from build123d import *

# Parameters (mm, degrees)
SKETCH1_W                = 457.2
SKETCH1_H                = 609.6
BOSS_EXTRUDE2_DEPTH      = 6.35
CUT_EXTRUDE1_REACH       = 764.026
SKETCH2_W                = 63.5
SKETCH2_H                = 68.58
SKETCH3_W                = 73.66
SKETCH3_H                = 27.94
CUT_EXTRUDE2_DEPTH       = 63.5
CUT_EXTRUDE4_DEPTH       = 763.026457874
CUT_EXTRUDE4_DEPTH_BACK  = 763.026457874
SKETCH5_W                = 5.08
SKETCH5_H                = 27.94
CUT_EXTRUDE5_DEPTH       = 763.026457874
CUT_EXTRUDE5_DEPTH_BACK  = 763.026457874
CUT_EXTRUDE6_DEPTH       = 763.026457874
CUT_EXTRUDE6_DEPTH_BACK  = 763.026457874
SKETCH7_W                = 12.7
SKETCH7_H                = 355.6
CUT_EXTRUDE8_START       = -6.35
CUT_EXTRUDE8_OUTLINE_W   = 6.35
CUT_EXTRUDE8_OUTLINE_H   = 127
CUT_EXTRUDE8_DEPTH       = 6.35
CUT_EXTRUDE9_DEPTH       = 763.026457874
CUT_EXTRUDE9_DEPTH_BACK  = 763.026457874
CUT_EXTRUDE10_START      = -6.35
CUT_EXTRUDE10_OUTLINE_W  = 6.35
CUT_EXTRUDE10_OUTLINE_H  = 127
CUT_EXTRUDE10_DEPTH      = 6.35
CUT_EXTRUDE11_DEPTH      = 759.233608461
CUT_EXTRUDE11_DEPTH_BACK = 759.233608461
CUT_EXTRUDE12_DEPTH      = 759.233608461
CUT_EXTRUDE12_DEPTH_BACK = 759.233608461
SKETCH4_R                = 6.4135
CUT_EXTRUDE13_DEPTH      = 759.233608461


# Read off the part's stored shape, not the designer's step: Cut-Extrude8, Cut-Extrude10
with BuildPart() as part:
    # Sketch1 → Boss-Extrude2 (new body)
    with BuildSketch(Plane.XY):
        with Locations((-228.6, 304.8)):
            Rectangle(SKETCH1_W, SKETCH1_H)
    extrude(amount=BOSS_EXTRUDE2_DEPTH)

    # Sketch2 → Cut-Extrude1 (cut, up to next)
    with BuildSketch(Plane.XY.offset(6.35), mode=Mode.PRIVATE) as cut_extrude1_sk1:
        with Locations((-111.175624359, 248.287614127)):
            Rectangle(SKETCH2_W, SKETCH2_H)
    cut_extrude1_tool1 = extrude(cut_extrude1_sk1.sketch, amount=-CUT_EXTRUDE1_REACH, mode=Mode.PRIVATE) & part.part
    add(cut_extrude1_tool1.solids().sort_by_distance((-111.175624, 248.287614, 6.35))[0], mode=Mode.SUBTRACT)

    # Sketch3 → Cut-Extrude2 (cut)
    with BuildSketch(Plane.XY.offset(6.35)):
        with Locations((-115.023623847, 327.440976048)):
            Rectangle(SKETCH3_W, SKETCH3_H)
    extrude(amount=-CUT_EXTRUDE2_DEPTH, mode=Mode.SUBTRACT)

    # Sketch5 → Cut-Extrude4 (cut, two sides: drawn at the far end of the back side and taken through both)
    with BuildSketch(Plane.XY.offset(6.35).offset(-CUT_EXTRUDE4_DEPTH_BACK)):
        with Locations((-75.653623847, 327.440976048)):
            Rectangle(SKETCH5_W, SKETCH5_H)
    extrude(amount=CUT_EXTRUDE4_DEPTH + CUT_EXTRUDE4_DEPTH_BACK, mode=Mode.SUBTRACT)

    # Sketch6 → Cut-Extrude5 (cut, two sides: drawn at the far end of the back side and taken through both)
    with BuildSketch(Plane.XY.offset(6.35).offset(-CUT_EXTRUDE5_DEPTH_BACK)):
        Polygon((-1796.763236556, 127), (-457.2, 127), (-444.5, 127), (-444.5, 482.6), (-457.2, 482.6), (-1796.763236556, 482.6), (-4475.889709667, 482.6), (-4475.889709667, 127), align=None)
    extrude(amount=CUT_EXTRUDE5_DEPTH + CUT_EXTRUDE5_DEPTH_BACK, mode=Mode.SUBTRACT)

    # Sketch7 → Cut-Extrude6 (cut, two sides: drawn at the far end of the back side and taken through both)
    with BuildSketch(Plane.XY.offset(6.35).offset(-CUT_EXTRUDE6_DEPTH_BACK)):
        with Locations((-6.35, 304.8)):
            Rectangle(SKETCH7_W, SKETCH7_H)
    extrude(amount=CUT_EXTRUDE6_DEPTH + CUT_EXTRUDE6_DEPTH_BACK, mode=Mode.SUBTRACT)

    # Cut-Extrude8 outline → Cut-Extrude8 (cut)
    with BuildSketch(Plane.XY.offset(6.35).offset(CUT_EXTRUDE8_START)):
        with Locations((-454.025, 63.5)):
            Rectangle(CUT_EXTRUDE8_OUTLINE_W, CUT_EXTRUDE8_OUTLINE_H)
    extrude(amount=CUT_EXTRUDE8_DEPTH, mode=Mode.SUBTRACT)

    # Sketch13 → Cut-Extrude9 (cut, two sides: drawn at the far end of the back side and taken through both)
    with BuildSketch(Plane.XY.offset(6.35).offset(-CUT_EXTRUDE9_DEPTH_BACK)):
        Polygon((-450.85, 2136.014036469), (-450.85, 609.6), (-450.85, 482.6), (-450.85, -1043.814036469), (-3503.678072938, -1043.814036469), (-3503.678072938, 2136.014036469), align=None)
    extrude(amount=CUT_EXTRUDE9_DEPTH + CUT_EXTRUDE9_DEPTH_BACK, mode=Mode.SUBTRACT)

    # Cut-Extrude10 outline → Cut-Extrude10 (cut)
    with BuildSketch(Plane.XY.offset(6.35).offset(CUT_EXTRUDE10_START)):
        with Locations((-3.175, 546.1)):
            Rectangle(CUT_EXTRUDE10_OUTLINE_W, CUT_EXTRUDE10_OUTLINE_H)
    extrude(amount=CUT_EXTRUDE10_DEPTH, mode=Mode.SUBTRACT)

    # Sketch16 → Cut-Extrude11 (cut, two sides: drawn at the far end of the back side and taken through both)
    with BuildSketch(Plane.XY.offset(6.35).offset(-CUT_EXTRUDE11_DEPTH_BACK)):
        Polygon((-6.35, 1645.896828812), (-6.35, 127), (-6.35, 0), (-6.35, -1518.896828812), (3031.443657625, -1518.896828812), (3031.443657625, 1645.896828812), align=None)
    extrude(amount=CUT_EXTRUDE11_DEPTH + CUT_EXTRUDE11_DEPTH_BACK, mode=Mode.SUBTRACT)

    # Sketch9 → Cut-Extrude12 (cut, two sides: drawn at the far end of the back side and taken through both)
    with BuildSketch(Plane.XY.offset(6.35).offset(-CUT_EXTRUDE12_DEPTH_BACK)):
        Polygon((-171.45, -1351.158484296), (-171.45, 0), (-171.45, 6.35), (-285.75, 6.35), (-285.75, 0), (-285.75, -1351.158484296), (-285.75, -4053.475452889), (-171.45, -4053.475452889), align=None)
    extrude(amount=CUT_EXTRUDE12_DEPTH + CUT_EXTRUDE12_DEPTH_BACK, mode=Mode.SUBTRACT)

    # Sketch4 → Cut-Extrude13 (cut, through all)
    with BuildSketch(Plane.XY.offset(6.35)):
        with Locations((-292.1, 516.89)):
            Circle(SKETCH4_R)
    extrude(amount=-CUT_EXTRUDE13_DEPTH, mode=Mode.SUBTRACT)


solid = part.part
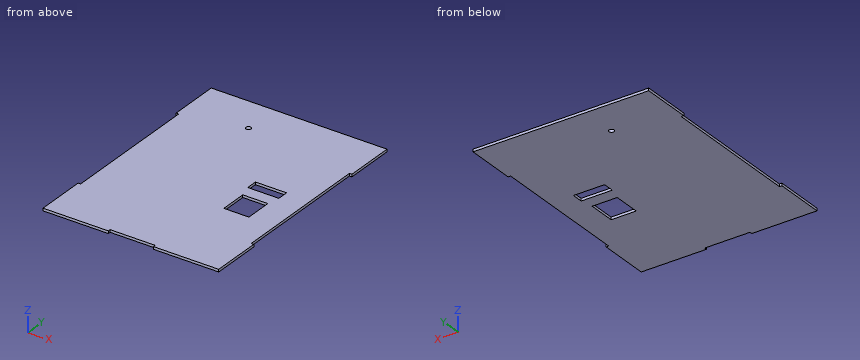
Check sheet for the modelled part. Datum: model origin and axes. Units: mm. Give positions to 0.01 mm unless a question says otherwise; leave off trailing zeros. Loops run counter-clockwise (first coordinate to the right, second up) from the corner with the lowest first, then second, coordinate; pieces in that order, holes last. Notation, with made-up numbers: M 46.25,30.25 L 55.25,30.25 A18 ccw 55.25,63.25 Z; hole C 29.5,-23 d5. An arc over 180 degrees is marked long. Return JSON: item names as keys, results as strings. Group by question number.
1. Go/stop test with flat-tipped pins: pin 1 (3 mm diameter, centred on y = 363, z = 1.5, fed in from +X); pin 2 (1.9 mm diameter, centred on y = 353, z = 4, fed in from -X); pin 3 (1.9 mm diameter, centred on x = -225.5, z = 3, fed in from -Y). Record where each tip stops, or that it passes through.
2. Cross-section at C-C on z = 5. Record the boundary of the cut face in (x, y), plus the area to 3 significant figures.
3. Cross-section at B-B on y = 223. Record the boundary of the cut face in (x, z), plus the area to 3 significant figures.
4. Cross-section at A-A on x = -292.1. Record the boundary of the cut face in (y, z), plus the area to 3 significant figures.
5. Thickness scan on L1, parallel to X at y = 516.89, z = 4.5; L2, parallel to Y at x = -292.1, z = 3; L3, parallel to X at y = 268, z = 2.5. Record the ranges inside material, lowest first.
Return value:
{
 "1": {"pin 1": "x = -12.7", "pin 2": "x = -444.5", "pin 3": "y = 6.35"},
 "2": {"outline": "M -450.85,0 L -285.75,0 L -285.75,6.35 L -171.45,6.35 L -171.45,0 L -6.35,0 L -6.35,127 L -12.7,127 L -12.7,482.6 L -6.35,482.6 L -6.35,609.6 L -450.85,609.6 L -450.85,482.6 L -444.5,482.6 L -444.5,127 L -450.85,127 Z; hole C -292.1,516.89 d12.83; hole M -151.85,313.47 L -73.11,313.47 L -73.11,341.41 L -151.85,341.41 Z; hole M -142.93,214 L -79.43,214 L -79.43,282.58 L -142.93,282.58 Z", "area": "259,000 mm^2"},
 "3": {"outline": "M -444.5,0 L -142.93,0 L -142.93,6.35 L -444.5,6.35 Z; M -79.43,0 L -12.7,0 L -12.7,6.35 L -79.43,6.35 Z", "area": "2,340 mm^2"},
 "4": {"outline": "M 0,0 L 510.48,0 L 510.48,6.35 L 0,6.35 Z; M 523.3,0 L 609.6,0 L 609.6,6.35 L 523.3,6.35 Z", "area": "3,790 mm^2"},
 "5": {"L1": "-450.85 to -298.51, -285.69 to -6.35", "L2": "0 to 510.48, 523.3 to 609.6", "L3": "-444.5 to -142.93, -79.43 to -12.7"}
}
